```python
from build123d import *

# Parameters (mm, degrees)
BOSS_EXTRUDE1_DEPTH = 850
SHELL1_T            = -2
SKETCH2_R           = 4
CUT_EXTRUDE1_DEPTH  = 851.730122418


with BuildPart() as part:
    # Sketch1 → Boss-Extrude1 (new body)
    with BuildSketch(Plane(origin=(0, 0, 0), x_dir=(1, 0, 0), z_dir=(0, 1, 0))):
        with BuildLine():
            Line((-24.801960973, -12), (24.801960973, -12))
            ThreePointArc((24.801960973, -12), (25.732910309, -11.365148372), (25.481830241, -10.266666667))
            ThreePointArc((25.481830241, -10.266666667), (21, 0), (25.481830241, 10.266666667))
            ThreePointArc((25.481830241, 10.266666667), (25.732910309, 11.365148372), (24.801960973, 12))
            Line((24.801960973, 12), (-24.801960973, 12))
            ThreePointArc((-24.801960973, 12), (-25.732910309, 11.365148372), (-25.481830241, 10.266666667))
            ThreePointArc((-25.481830241, 10.266666667), (-21, 0), (-25.481830241, -10.266666667))
            ThreePointArc((-25.481830241, -10.266666667), (-25.732910309, -11.365148372), (-24.801960973, -12))
        make_face()
    extrude(amount=BOSS_EXTRUDE1_DEPTH)

    # Shell1
    shell1_openings = [part.faces().sort_by_distance(p)[0] for p in [
        (0, 850, 0),
        (0, 0, 0),
    ]]
    offset(amount=SHELL1_T, openings=shell1_openings, kind=Kind.INTERSECTION)

    # Sketch2 → Cut-Extrude1 (cut, through all)
    with BuildSketch(Plane(origin=(0, 0, -12), x_dir=(-1, 0, 0), z_dir=(0, 0, -1))):
        with Locations((0, 755)):
            Circle(SKETCH2_R)
    extrude(amount=-CUT_EXTRUDE1_DEPTH, mode=Mode.SUBTRACT)


solid = part.part
```
CAD build for the part. Positions are in the model's coordinates, mm. Round coordinates to 2 decimals unless told otherwise and drop trailing zeros. Order: outer loops, then holes, each group sorted by start corner. A loop starts at its lowest first (then second) coordinate and runs counter-clockwise, first axis right, second up. Notation, with made-up numbers: (3.25, -34) - (45.25, -34) arc R29 cw to (45.25, 1) - close; hole circle Ø9 at (23.25, 21). An arc over 180 degrees is marked (long way). Answer as CSV lines item,"result". Start each with the question number.
1. Pull direction X, two halves, no side cores. Call faces 1 (the face through (0, 419, -10)), 2 (the face through (21, 419, 0)), 3 (the face through (0, 0, 11)): +X half, -X half, draft (parallel to the pull), parting line (faces both ways), or undercut.
2. Pin check, flat tips, straight feed: pin 1 (12 mm diameter, centred on y = 229, z = -4.5, fed in from -X); pin 2 (3 mm diameter, centred on y = 626, z = 8.5, fed in from +X); pin 3 (5 mm diameter, centred on x = 0, y = 755, fed in from -Z) (3 decimals). Stop position of each tip, or through.
3. Drill centre lines: L1, parallel to X at y = 755, z = -10.5; L2, parallel to Z at x = -1, y = 272; L3, parallel to X at y = 61, z = 0.5. Where is each one in solid material? Low to high. Write a range as [from, to].
4. Saw through at A-A, the plane y = 575. Write the cut outline in (x, z).
5. Saw through at B-B, the plane z = -5.25. Write the cut outline in (x, y), and give its area (3 significant figures).
Model answer:
1,face 1,"undercut"
1,face 2,"+X half"
1,face 3,"draft"
2,pin 1,"stops at x = -25.67"
2,pin 2,"stops at x = 25.2"
2,pin 3,"passes through"
3,L1,"x = [-25.67, -4], [4, 25.67]"
3,L2,"z = [-12, -10], [10, 12]"
3,L3,"x = [-21.01, -19.01], [19.01, 21.01]"
4,outline,"(-25.48, -10.27) arc R1 ccw to (-24.8, -12) - (24.8, -12) arc R1 ccw to (25.48, -10.27) arc R14 cw to (25.48, 10.27) arc R1 ccw to (24.8, 12) - (-24.8, 12) arc R1 ccw to (-25.48, 10.27) arc R14 cw to start; hole (-22.51, -10) - (22.51, -10) arc R16 cw to (22.51, 10) - (-22.51, 10) arc R16 cw to start"
5,outline,"(-22.02, 0) - (-19.89, 0) - (-19.89, 850) - (-22.02, 850) - close; (19.89, 0) - (22.02, 0) - (22.02, 850) - (19.89, 850) - close"
5,area,"3,630 mm²"
